```python
from build123d import *

# Parameters (mm, degrees)
ESQUISSE1_R        = 12.3
ESQUISSE1_R_2      = 1.97989757
ESQUISSE1_R_3      = 3
BOSS_EXTRU_1_DEPTH = 2
ESQUISSE2_R        = 12.3
ESQUISSE2_R_2      = 3.175426481
ESQUISSE2_R_3      = 3
BOSS_EXTRU_2_DEPTH = 2.5
ESQUISSE3_R        = 2.475
BOSS_EXTRU_3_DEPTH = 16


with BuildPart() as part:
    # Esquisse1 → Boss.-Extru.1 (new body)
    with BuildSketch(Plane.XY):
        Circle(ESQUISSE1_R)
        with Locations((-8.3, -0.297454923)):
            Circle(ESQUISSE1_R_2, mode=Mode.SUBTRACT)
        with Locations((-0.297454923, 8.3)):
            Circle(ESQUISSE1_R_2, mode=Mode.SUBTRACT)
        with Locations((8.3, 0.297454923)):
            Circle(ESQUISSE1_R_2, mode=Mode.SUBTRACT)
        with Locations((0.297454923, -8.3)):
            Circle(ESQUISSE1_R_2, mode=Mode.SUBTRACT)
        Circle(ESQUISSE1_R_3, mode=Mode.SUBTRACT)
    extrude(amount=BOSS_EXTRU_1_DEPTH)

    # Esquisse2 → Boss.-Extru.2 (add)
    # profile 1 of 2: a face of its own
    with BuildSketch(Plane.XY.offset(2)):
        Circle(ESQUISSE2_R)
        with Locations((0.297454923, -8.3)):
            Circle(ESQUISSE2_R_2, mode=Mode.SUBTRACT)
        with Locations((8.3, 0.297454923)):
            Circle(ESQUISSE2_R_2, mode=Mode.SUBTRACT)
        with Locations((-0.297454923, 8.3)):
            Circle(ESQUISSE2_R_2, mode=Mode.SUBTRACT)
        with Locations((-8.3, -0.297454923)):
            Circle(ESQUISSE2_R_2, mode=Mode.SUBTRACT)
        Circle(ESQUISSE2_R_3, mode=Mode.SUBTRACT)
    # profile 2 of 2: a face of its own
    with BuildSketch(Plane.XY.offset(2)):
        Circle(ESQUISSE2_R_3)
    extrude(amount=BOSS_EXTRU_2_DEPTH)

    # Esquisse3 → Boss.-Extru.3 (add)
    with BuildSketch(Plane.XY.offset(4.5)):
        Circle(ESQUISSE3_R)
    extrude(amount=BOSS_EXTRU_3_DEPTH)


solid = part.part
```
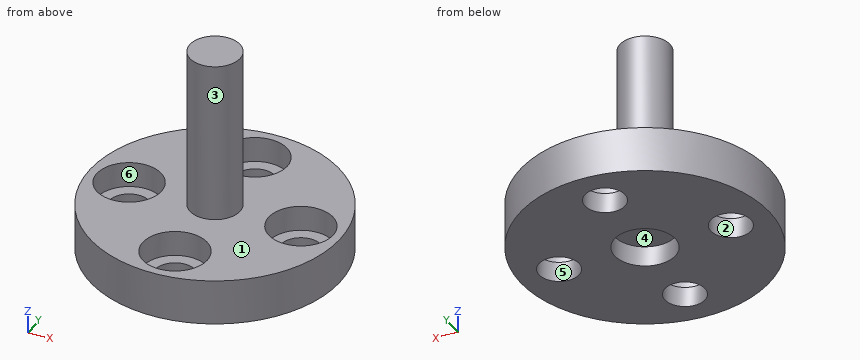
Model file for the job. Use its own axes, mm. Face numbers are marked on the shaded views. A direction names the side the tool comes from. Coordinates: 2 decimals unless noted, no trailing zeros. Write each loop counter-clockwise with the first axis right and the second up, starting at its lowest first coordinate (ties: lowest second). Pieces come first, ordered by that corner, then holes. Notation, with made-up numbers: (18, -38.75) - (47, -38.75) arc R19 cw to (47, -10.75) - close; hole circle Ø5 at (28, 74). An arc over 180 degrees is marked (long way). One line per item, written item: value. Start each with the question number.
1. Probe line 1 (Z direction, x = -7, y = 5.25); line 2 (Z direction, x = 0.75, y = 1); line 3 (X direction, y = -1.5, z = 3.5). List the from-to ranges inside material, lowest first. Write a range as from..to.
2. Slice it at D-D (z = 11.75). Write the cut outline in (x, y) (3 decimals).
3. Flat gauge pins, fed straight in: pin 1 (10 mm diameter, centred on x = -8.3, y = -0.3, fed in from +Z); pin 2 (3 mm diameter, centred on x = -1, z = 16.5, fed in from -Y) (3 decimals); pin 3 (6 mm diameter, centred on y = 5.5, z = 2, fed in from -X). Where does each tip first touch, or does it go through?
4. Tool access for the marked faces 4, 5 and 6: list every direction of +Z, -Z, +X, -X, +Y, -Y with a clear straight run to the whole face (end or side of a thin tool).
5. Slice it at A-A (x = 0). Write the cut outline in (y, z) (3 decimals), plus the area to 3 significant figures.
6. Slice it at C-C (y = 8.3). Write the cut outline in (x, z).
7. Mould opens along Y. For the marked faces 1, 2 and 3 say: released by +Y, released by -Y, zero draft, split by the parting line, or undercut.
8. Slice it at B-B (x = 7.5). Write the cut outline in (y, z), plus the area to 3 significant figures.
Answers below:
1. line 1: z = 0..4.5
1. line 2: z = 2..20.5
1. line 3: x = -12.21..-11.24, -5.36..5.68, 10.92..12.21
2. outline: circle Ø4.95 at (0, 0)
3. pin 1: stops at z = 4.5
3. pin 2: stops at y = -2.475
3. pin 3: stops at x = -12.04
4. face 4: -Z
4. face 5: +Z, -Z
4. face 6: +Z
5. outline: (-12.3, 0) - (-10.257, 0) - (-10.257, 2) - (-11.461, 2) - (-11.461, 4.5) - (-12.3, 4.5) - close; (-6.343, 0) - (-3, 0) - (-3, 2) - (3, 2) - (3, 0) - (6.343, 0) - (6.343, 2) - (5.139, 2) - (5.139, 4.5) - (2.475, 4.5) - (2.475, 20.5) - (-2.475, 20.5) - (-2.475, 4.5) - (-5.139, 4.5) - (-5.139, 2) - (-6.343, 2) - close; (10.257, 0) - (12.3, 0) - (12.3, 4.5) - (11.461, 4.5) - (11.461, 2) - (10.257, 2) - close
5. area: 131 mm^2
6. outline: (-9.08, 0) - (-2.28, 0) - (-2.28, 2) - (-3.47, 2) - (-3.47, 4.5) - (-9.08, 4.5) - close; (1.68, 0) - (9.08, 0) - (9.08, 4.5) - (2.88, 4.5) - (2.88, 2) - (1.68, 2) - close
7. face 1: zero draft
7. face 2: undercut
7. face 3: split by the parting line
8. outline: (-9.75, 0) - (-1.51, 0) - (-1.51, 2) - (-2.78, 2) - (-2.78, 4.5) - (-9.75, 4.5) - close; (2.11, 0) - (9.75, 0) - (9.75, 4.5) - (3.37, 4.5) - (3.37, 2) - (2.11, 2) - close
8. area: 65.1 mm^2
